```python
from build123d import *

# Parameters (mm, degrees)
BOSS_EXTRUDE1_DEPTH         = 11.90625
F_1_4_0_25_DIAMETER_HOLE1_D = 6.35


with BuildPart() as part:
    # Sketch1 → Boss-Extrude1 (new body)
    with BuildSketch(Plane(origin=(0, 0, 0), x_dir=(0, 0, -1), z_dir=(1, 0, 0))):
        Polygon((0, 0), (0, 254), (250.141169265, -44.106637127), align=None)
    extrude(amount=BOSS_EXTRUDE1_DEPTH)

    # 1/4 (0.25) Diameter Hole1 (through all)
    with Locations(Plane.ZY):
        with Locations((-44.45, 171.725527446), (-44.45, 108.225527446), (-63.236968779, 53.06211718), (-114.3, 24.981539003), (-176.835292316, 13.954879721)):
            Hole(F_1_4_0_25_DIAMETER_HOLE1_D / 2)


solid = part.part
```
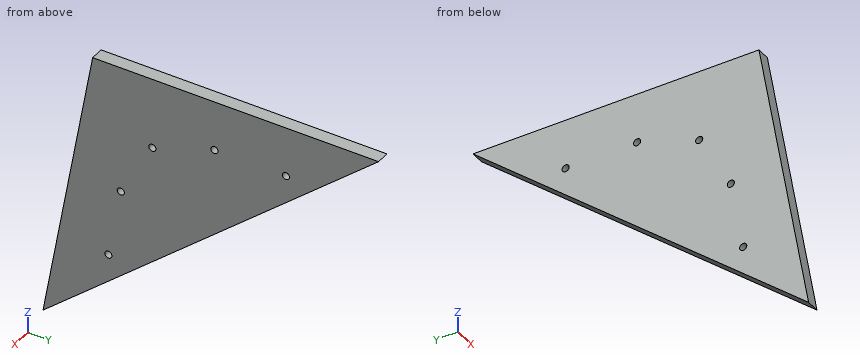
Geometry check sheet. Reference: the model listing, model coordinates, mm. Coordinates: 2 decimals unless noted, no trailing zeros. Order: outer loops, then holes, each group sorted by start corner. A loop starts at its lowest first (then second) coordinate and runs counter-clockwise, first axis right, second up. Notation, with made-up numbers: (-6.75, 72.5) - (11.25, 72.5) arc R33 ccw to (11.25, 110.5) - close; hole circle Ø4 at (-5.5, 81.25). An arc over 180 degrees is marked (long way). Answer in a Markdown table with one row per item. Add a question column.
1. Section check A-A (z = -44.45). Enter the section's corners in (x, y), plus the area to 3 significant figures.
2. Section check B-B (x = 5.25). Enter the section's corners in (y, z) (3 decimals).
3. Material ranges on L1, parallel to Y at x = 3.25, z = -44.45; L2, parallel to Y at x = 10, z = -44; L3, parallel to Y at x = 6, z = -114.3, recorded low to high. Write a range as [from, to].
4. Section check C-C (z = -114.3). Enter the section's corners in (x, y).
5. Section check D-D (y = 40). Enter the section's corners in (x, z), plus the area to 3 significant figures.
6. Gauge pin test, flat ends, axial feed: pin 1 Ø4 at (x, z) = (4.5, -174.5) entering from -Y; pin 2 Ø1 at (x, y) = (8.5, 40.5) entering from -Z; pin 3 Ø4 at (x, y) = (2.5, 165.5) entering from -Z. Record the tip position at first contact, or that the pin passes through.
Data:
| question | item | result |
|---|---|---|
| 1 | outline | (0, -7.84) - (11.91, -7.84) - (11.91, 105.05) - (0, 105.05) - close; (0, 111.4) - (11.91, 111.4) - (11.91, 168.55) - (0, 168.55) - close; (0, 174.9) - (11.91, 174.9) - (11.91, 201.03) - (0, 201.03) - close |
| 1 | area | 2,340 mm² |
| 2 | outline | (-44.107, -250.141) - (254, 0) - (0, 0) - close; hole circle Ø6.35 at (13.955, -176.835); hole circle Ø6.35 at (24.982, -114.3); hole circle Ø6.35 at (53.062, -63.237); hole circle Ø6.35 at (108.226, -44.45); hole circle Ø6.35 at (171.726, -44.45) |
| 3 | L1 | y = [-7.84, 105.05], [111.4, 168.55], [174.9, 201.03] |
| 3 | L2 | y = [-7.76, 105.08], [111.37, 168.58], [174.87, 201.56] |
| 3 | L3 | y = [-20.15, 21.81], [28.16, 117.78] |
| 4 | outline | (0, -20.15) - (11.91, -20.15) - (11.91, 21.81) - (0, 21.81) - close; (0, 28.16) - (11.91, 28.16) - (11.91, 117.78) - (0, 117.78) - close |
| 5 | outline | (0, -179.57) - (11.91, -179.57) - (11.91, 0) - (0, 0) - close |
| 5 | area | 2,140 mm² |
| 6 | pin 1 | stops at y = -31.12 |
| 6 | pin 2 | stops at z = -179.57 |
| 6 | pin 3 | stops at z = -75.94 |
